CAD build for the part. Positions are in the model's coordinates, mm. A direction names the side the tool comes from. Round coordinates to 2 decimals unless told otherwise and drop trailing zeros. Loops run counter-clockwise (first coordinate to the right, second up) from the corner with the lowest first, then second, coordinate; pieces in that order, holes last.
```python
from build123d import *

# Parameters (mm, degrees)
F0_R      = 3.5
F0_R_2    = 25.4
F1_DEPTH  = 5.5
F2_DEPTH  = 33
F3_DEPTH  = 28
F4_R      = 2.5
F5_DEPTH  = 25.4
F6_R      = 5.08
F7_R      = 40.64
F8_DEPTH  = 33
F9_R      = 1.7526
F10_DEPTH = 5.501


with BuildPart() as f1:
    # F0 (on Top) → F1 (new body)
    with BuildSketch(Plane.XY):
        with BuildLine():
            Line((-3.3917498572, 9.4072330101), (-2.8084065037, 9.5975441082))
            ThreePointArc((-2.8084065037, 9.5975441082), (-3.1015382157, 9.5068638728), (-3.3917498572, 9.4072330101))
        make_face()
        with BuildLine():
            Line((35.7055754428, 22.1624223313), (-2.8084065037, 9.5975441082))
            Line((-2.8084065037, 9.5975441082), (-3.3917498572, 9.4072330101))
            ThreePointArc((-3.3917498572, 9.4072330101), (-9.9089012804, 1.3467276694), (-5.7794328291, -8.1607693371))
            Line((-5.7794328291, -8.1607693371), (28.3037582299, -32.2983849452))
            ThreePointArc((28.3037582299, -32.2983849452), (15.5024060308, -2.8251442248), (35.7055754428, 22.1624223313))
        make_face()
        Circle(F0_R, mode=Mode.SUBTRACT)
        with BuildLine():
            ThreePointArc((55.9525424009, 22.43259449), (45.80637798, 23.9972404711), (35.7055754428, 22.1624223313))
            ThreePointArc((35.7055754428, 22.1624223313), (15.5024060308, -2.8251442248), (28.3037582299, -32.2983849452))
            ThreePointArc((28.3037582299, -32.2983849452), (46.3284941146, -37.999810145), (64.3128808741, -32.1723590805))
            ThreePointArc((64.3128808741, -32.1723590805), (73.805134648, -21.1442690321), (77.22, -7))
            ThreePointArc((77.22, -7), (71.3467667481, 11.1561447666), (55.9525424009, 22.43259449))
        make_face()
        with Locations((46.22, -7)):
            Circle(F0_R_2, mode=Mode.SUBTRACT)
        with BuildLine():
            Line((95.0795298067, 9.4943853194), (55.9525424009, 22.43259449))
            ThreePointArc((55.9525424009, 22.43259449), (71.3467667481, 11.1561447666), (77.22, -7))
            ThreePointArc((77.22, -7), (73.805134648, -21.1442690321), (64.3128808741, -32.1723590805))
            Line((64.3128808741, -32.1723590805), (97.7764131852, -8.1201158324))
            ThreePointArc((97.7764131852, -8.1201158324), (101.8248141538, 1.5134229894), (95.0795298067, 9.4943853194))
        make_face()
        with BuildLine():
            ThreePointArc((91.44, -3.5), (87.94, 0), (91.44, 3.5))
            Line((91.44, 3.5), (92.44, 3.5))
            ThreePointArc((92.44, 3.5), (95.94, 0), (92.44, -3.5))
            Line((92.44, -3.5), (91.44, -3.5))
        make_face(mode=Mode.SUBTRACT)
    extrude(amount=F1_DEPTH)

    # F0 (on Top) → F2 (join)
    with BuildSketch(Plane.XY):
        with BuildLine():
            ThreePointArc((55.9525424009, 22.43259449), (45.80637798, 23.9972404711), (35.7055754428, 22.1624223313))
            ThreePointArc((35.7055754428, 22.1624223313), (15.5024060308, -2.8251442248), (28.3037582299, -32.2983849452))
            ThreePointArc((28.3037582299, -32.2983849452), (46.3284941146, -37.999810145), (64.3128808741, -32.1723590805))
            ThreePointArc((64.3128808741, -32.1723590805), (73.805134648, -21.1442690321), (77.22, -7))
            ThreePointArc((77.22, -7), (71.3467667481, 11.1561447666), (55.9525424009, 22.43259449))
        make_face()
        with Locations((46.22, -7)):
            Circle(F0_R_2, mode=Mode.SUBTRACT)
        with Locations((46.22, -7)):
            Circle(F0_R_2)
    extrude(amount=-F2_DEPTH)

    # F0 (on Top) → F3 (cut)
    with BuildSketch(Plane.XY):
        with Locations((46.22, -7)):
            Circle(F0_R_2)
    extrude(amount=-F3_DEPTH, mode=Mode.SUBTRACT)

    # F4 (on face) → F5 (cut)
    with BuildSketch(Plane(origin=(0, 0, -33), x_dir=(1, 0, 0), z_dir=(0, 0, -1))):
        with Locations((46.22, 7)):
            Circle(F4_R)
    extrude(amount=-F5_DEPTH, mode=Mode.SUBTRACT)

    # F6
    f6_edges = [f1.edges().sort_by_distance(p)[0] for p in [
        (36.487458, -36.432594, -33),
    ]]
    fillet(f6_edges, radius=F6_R)

    # F7 (on face) → F8 (cut, through all)
    with BuildSketch(Plane(origin=(0, 0, -33), x_dir=(1, 0, 0), z_dir=(0, 0, -1))):
        with Locations((46.22, 7)):
            Circle(F7_R)
    extrude(amount=-F8_DEPTH, mode=Mode.SUBTRACT)

    # F9 (on face) → F10 (cut, through all)
    with BuildSketch(Plane.XY.offset(5.5)):
        with Locations((26.3511833321, 12.8688166679)):
            Circle(F9_R)
        with Locations((26.3511833321, -26.8688166679)):
            Circle(F9_R)
        with Locations((66.0888166679, -26.8688166679)):
            Circle(F9_R)
        with Locations((66.0888166679, 12.8688166679)):
            Circle(F9_R)
    extrude(amount=-F10_DEPTH, mode=Mode.SUBTRACT)


solid = f1.part
```
Item 1: 3-axis set-ups, long thin cutter, end or side, ignore diameter. For faces 5 (the cylindrical face through (87.94, -0.08, 2.71)), 6 (the cylindrical face through (46, -38, 3)): which of +Z, -Z, +X, -X, +Y, -Y reach the whole face in a straight line?
Answers follow:
face 5: +Z, -Z
face 6: +Z, -Z, -Y
Item 2: Two-plate mould, pull along X, no slides. Class faces 1 (the cylindrical face through (27.5, 10.17, 2.71)), 2 (the cylindrical face through (3.233, -1.341, 2.712)), 3 (the flat face through (80.81, -20.315, 2.712)), 4 (the flat face through (33, 16, 5.5)): released by +X, released by -X, zero draft, split by the parting line, or undercut.
Answers follow:
face 1: undercut
face 2: undercut
face 3: released by +X
face 4: zero draft
Item 3: Cut at D-D, the plane z = 2.35. Give the cut face in (x, y), plus the area to 3 significant figures.
Answers follow:
outline: (-5.78, -8.16) - (28.3, -32.3) arc R31 ccw to (64.31, -32.17) - (97.78, -8.12) arc R10 ccw to (95.08, 9.49) - (55.95, 22.43) arc R31 ccw to (35.71, 22.16) - (-2.81, 9.6) arc R10 ccw to start; hole circle Ø7 at (0, 0); hole circle Ø50.8 at (46.22, -7); hole circle Ø3.51 at (26.35, -26.87); hole circle Ø3.51 at (26.35, 12.87); hole circle Ø3.51 at (66.09, -26.87); hole circle Ø3.51 at (66.09, 12.87); hole (91.44, -3.5) - (92.44, -3.5) arc R3.5 ccw to (92.44, 3.5) - (91.44, 3.5) arc R3.5 ccw to start
area: 2,370 mm2
Item 4: Cut at B-B, the plane x = 46.22. Give the cut face in (y, z).
Answers follow:
outline: (-38, 0) - (-32.4, 0) - (-32.4, 5.5) - (-38, 5.5) - close; (18.4, 0) - (24, 0) - (24, 5.5) - (18.4, 5.5) - close
Item 5: Cut at A-A, the plane y = -7. Give the cut face in (x, z), plus the area to 3 significant figures.
Answers follow:
outline: (-7.14, 0) - (20.82, 0) - (20.82, 5.5) - (-7.14, 5.5) - close; (71.62, 0) - (99.08, 0) - (99.08, 5.5) - (71.62, 5.5) - close
area: 305 mm2
Item 6: Probe line 1 (X direction, y = -1, z = 0.65); line 2 (X direction, y = 0.5, z = 3.3); line 3 (Y direction, x = 47, z = 0.6). List the from-to ranges inside material, lowest first.
Answers follow:
line 1: x = -9.95 to -3.35, 3.35 to 21.54, 70.9 to 88.09, 95.79 to 101.89
line 2: x = -9.99 to -3.46, 3.46 to 21.95, 70.49 to 87.98, 95.9 to 101.93
line 3: y = -37.99 to -32.39, 18.39 to 23.99
Item 7: Cut at C-C, the plane y = 0. Give the cut face in (x, z).
Answers follow:
outline: (-10, 0) - (-3.5, 0) - (-3.5, 5.5) - (-10, 5.5) - close; (3.5, 0) - (21.8, 0) - (21.8, 5.5) - (3.5, 5.5) - close; (70.64, 0) - (87.94, 0) - (87.94, 5.5) - (70.64, 5.5) - close; (95.94, 0) - (101.94, 0) - (101.94, 5.5) - (95.94, 5.5) - close
Item 8: Flat gauge pins, fed straight in: P1, Ø1, axis at y = -22, z = 2, coming from the -X side; P2, Ø1.1, axis at x = 92, z = 3.5, coming from the -Y side; P3, Ø1, axis at x = 23, z = 4.5, coming from the -Y side. Where does each tip first touch, or does it go through?
Answers follow:
P1: stops at x = 13.06
P2: stops at y = -12.67
P3: stops at y = -28.9
